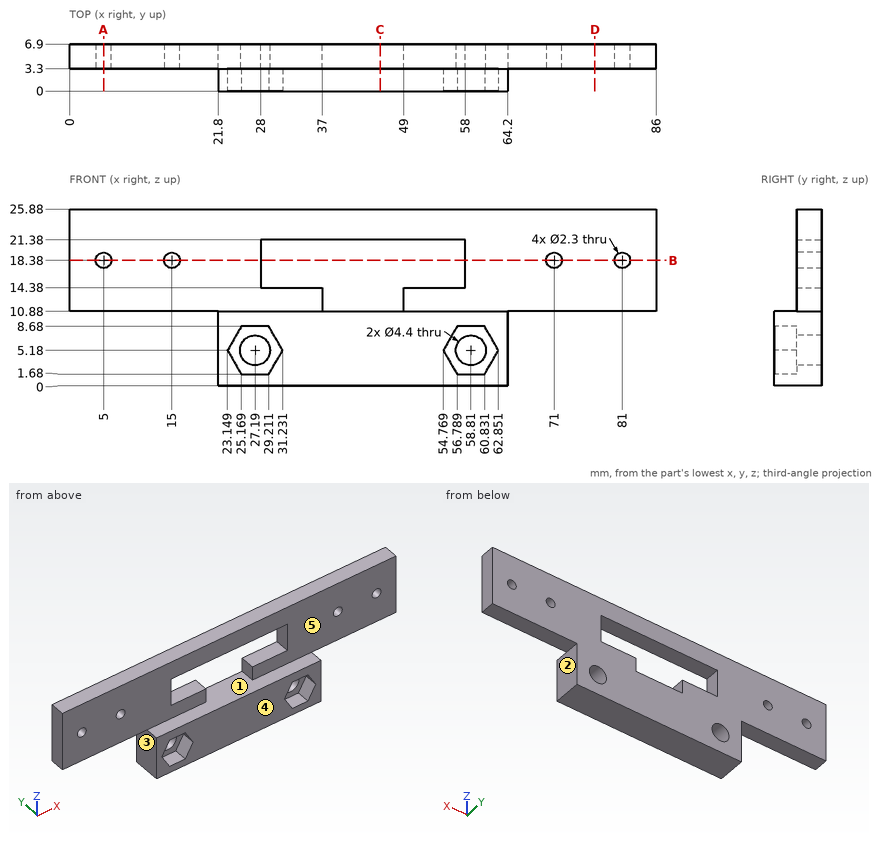
Part print with two shaded views. Sizes in mm from the minimum x, y, z corner. A direction names the side the tool comes from. Round coordinates to 2 decimals unless told otherwise and drop trailing zeros. Loops run counter-clockwise (first coordinate to the right, second up) from the corner with the lowest first, then second, coordinate; pieces in that order, holes last. Notation, with made-up numbers: (-31.5, 63.5) - (-10.5, 63.5) arc R15 ccw to (-10.5, 69.5) - close; hole circle Ø7 at (18.5, 15.25). An arc over 180 degrees is marked (long way). Answer as a JSON object with one key per item and string values.
Item 1: Pin check, flat tips, straight feed: pin 1 (2.5 mm diameter, centred on x = 28, y = 2, fed in from -Z); pin 2 (3.5 mm diameter, centred on y = 3, z = 4.5, fed in from -X); pin 3 (2 mm diameter, centred on y = 2, z = 6, fed in from +X); pin 4 (1.1 mm diameter, centred on x = 71, y = 4.5, fed in from -Z). Stop position of each tip, or through.
Output:
{"pin 1": "z = 0", "pin 2": "x = 21.8", "pin 3": "x = 64.2", "pin 4": "z = 10.88"}
Item 2: Band-saw the part on D-D on x = 77. List the corners of the cut face in (y, z), plus the area to 3 significant figures.
Output:
{"outline": "(3.3, 10.88) - (6.9, 10.88) - (6.9, 25.88) - (3.3, 25.88) - close", "area": "54.0 mm2"}
Item 3: Wall check: L1, parallel to X at y = 4.1, z = 5.18; L2, parallel to X at y = 6.05, z = 18.38; L3, parallel to Z at x = 27.19, y = 5.8. Give the ranges that are in metal, low to high.
Output:
{"L1": "21.8 to 24.99, 29.39 to 56.61, 61.01 to 64.2", "L2": "0 to 3.85, 6.15 to 13.85, 16.15 to 28, 58 to 69.85, 72.15 to 79.85, 82.15 to 86", "L3": "0 to 2.98, 7.38 to 25.88"}
Item 4: Tool access for the marked faces 4 and 5: list every direction of +Z, -Z, +X, -X, +Y, -Y with a clear straight run to the whole face (end or side of a thin tool).
Output:
{"face 4": "+Z, -Z, +X, -X, -Y", "face 5": "+Z, +X, -X, -Y"}
Item 5: Band-saw the part on A-A on x = 5. List the corners of the cut face in (y, z).
Output:
{"outline": "(3.3, 10.88) - (6.9, 10.88) - (6.9, 17.23) - (3.3, 17.23) - close; (3.3, 19.53) - (6.9, 19.53) - (6.9, 25.88) - (3.3, 25.88) - close"}
Item 6: Band-saw the part on B-B on z = 18.38. List the corners of the cut face in (x, y).
Output:
{"outline": "(0, 3.3) - (3.85, 3.3) - (3.85, 6.9) - (0, 6.9) - close; (6.15, 3.3) - (13.85, 3.3) - (13.85, 6.9) - (6.15, 6.9) - close; (16.15, 3.3) - (28, 3.3) - (28, 6.9) - (16.15, 6.9) - close; (58, 3.3) - (69.85, 3.3) - (69.85, 6.9) - (58, 6.9) - close; (72.15, 3.3) - (79.85, 3.3) - (79.85, 6.9) - (72.15, 6.9) - close; (82.15, 3.3) - (86, 3.3) - (86, 6.9) - (82.15, 6.9) - close"}
Item 7: Pull direction X, two halves, no side cores. Call the marked faces 1, 2 and 3: pulls with the +X half, pulls with the -X half, needs draft (parallel to the pull), parting line crosses it, or undercut.
Output:
{"face 1": "undercut", "face 2": "pulls with the +X half", "face 3": "pulls with the -X half"}
Item 8: Band-saw the part on C-C on x = 45.5. List the corners of the cut face in (y, z).
Output:
{"outline": "(0, 0) - (6.9, 0) - (6.9, 10.88) - (0, 10.88) - close; (3.3, 21.38) - (6.9, 21.38) - (6.9, 25.88) - (3.3, 25.88) - close"}
